Part print with two shaded views. Sizes in mm from the minimum x, y, z corner. Round coordinates to 2 decimals unless told otherwise and drop trailing zeros. Write each loop counter-clockwise with the first axis right and the second up, starting at its lowest first coordinate (ties: lowest second). Pieces come first, ordered by that corner, then holes. Notation, with made-up numbers: (-8, 3.25) -> (28, 3.25) arc R15 ccw to (28, 29.25) -> close; hole circle Ø9 at (57, 2). An arc over 180 degrees is marked (long way). Answer in a Markdown table with one row per item.
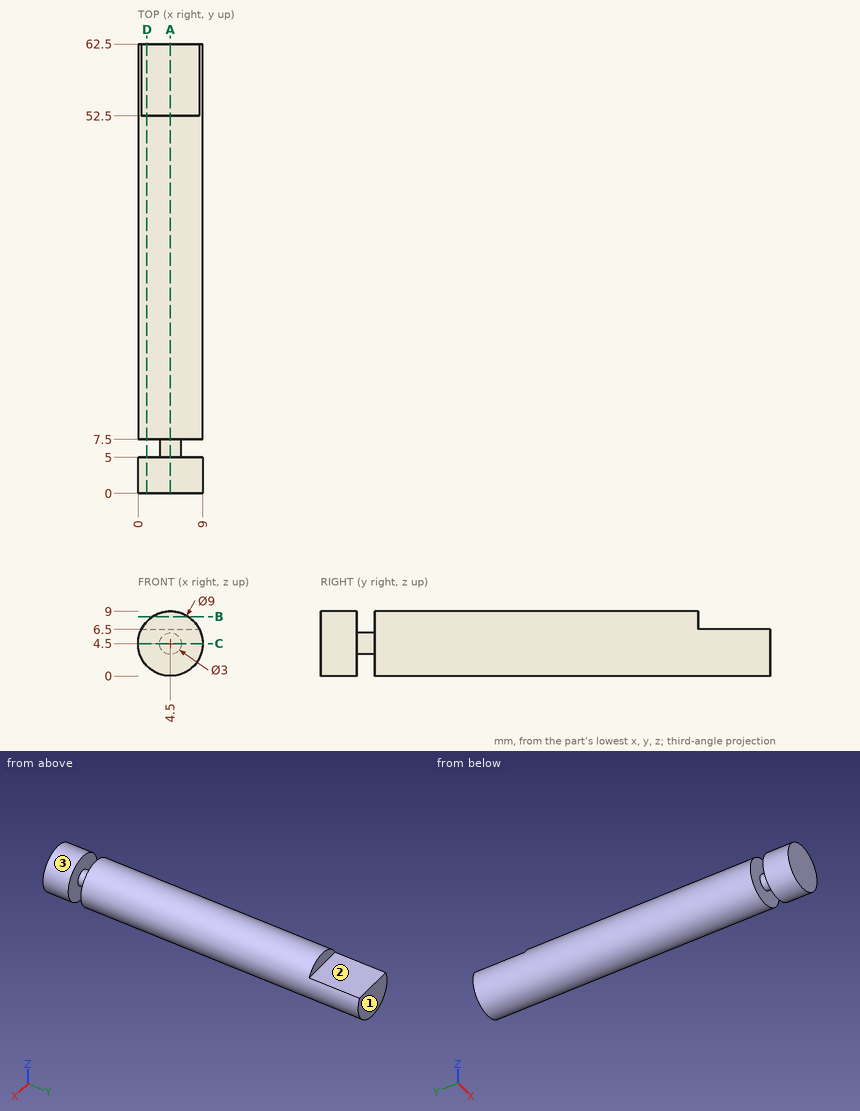
Q1. Two-plate mould, pull along Z, no slides. Class the marked faces 1, 2 and 3: released by +Z, released by -Z, zero draft, split by the parting line, or undercut.
A:
| item | result |
|---|---|
| face 1 | zero draft |
| face 2 | released by +Z |
| face 3 | split by the parting line |
Q2. Saw through at D-D on x = 1.25. Write the cut outline in (y, z), plus the area to 3 significant figures.
A:
| item | result |
|---|---|
| outline | (0, 1.39) -> (5, 1.39) -> (5, 7.61) -> (0, 7.61) -> close; (7.5, 1.39) -> (62.5, 1.39) -> (62.5, 6.5) -> (52.5, 6.5) -> (52.5, 7.61) -> (7.5, 7.61) -> close |
| area | 362 mm² |
Q3. Saw through at B-B on z = 8.25. Write the cut outline in (x, y).
A:
| item | result |
|---|---|
| outline | (2.01, 0) -> (6.99, 0) -> (6.99, 5) -> (2.01, 5) -> close; (2.01, 7.5) -> (6.99, 7.5) -> (6.99, 52.5) -> (2.01, 52.5) -> close |
Q4. Saw through at C-C on z = 4.5. Write the cut outline in (x, y).
A:
| item | result |
|---|---|
| outline | (0, 0) -> (9, 0) -> (9, 5) -> (6, 5) -> (6, 7.5) -> (9, 7.5) -> (9, 62.5) -> (0, 62.5) -> (0, 7.5) -> (3, 7.5) -> (3, 5) -> (0, 5) -> close |
Q5. Drop flat-ended pins along their axis: P1, Ø1, axis at x = 8, y = 38.5, coming from the +Z side; P2, Ø4.5, axis at x = 6, z = 2.5, coming from the -Y side; P3, Ø0.8, axis at x = 3.5, z = 7.5, coming from the +Y side; P4, Ø5, axis at y = 13.5, z = 7.5, coming from the +X side. Give the stop position or say it passes through.
A:
| item | result |
|---|---|
| P1 | z = 7.85 |
| P2 | y = 0 |
| P3 | y = 52.5 |
| P4 | x = 8.97 |
Q6. Saw through at A-A on x = 4.5. Write the cut outline in (y, z).
A:
| item | result |
|---|---|
| outline | (0, 0) -> (5, 0) -> (5, 3) -> (7.5, 3) -> (7.5, 0) -> (62.5, 0) -> (62.5, 6.5) -> (52.5, 6.5) -> (52.5, 9) -> (7.5, 9) -> (7.5, 6) -> (5, 6) -> (5, 9) -> (0, 9) -> close |
Q7. Wall check: line 1 (Y direction, x = 4, z = 2.25); line 2 (Y direction, x = 5.5, z = 7.75); line 3 (Z direction, x = 2.5, y = 44). Give the ranges that are in metal, low to high. Write a range as [from, to].
A:
| item | result |
|---|---|
| line 1 | [0, 5], [7.5, 62.5] |
| line 2 | [0, 5], [7.5, 52.5] |
| line 3 | [0.47, 8.53] |
